from build123d import *

# Parameters (mm, degrees)
EXTRUDE_1_DEPTH = 35
FILLET_1_R      = 3


with BuildPart() as part:
    # 스케치1 → 보스-돌출1 (new body)
    with BuildSketch(Plane.XY):
        with BuildLine():
            Line((0, 0), (52.851450041, 0))
            Line((52.851450041, 0), (25.161162212, 33))
            ThreePointArc((25.161162212, 33), (20.274657466, 29.059278699), (15.388152719, 33))
            Line((15.388152719, 33), (0, 0))
        make_face()
    extrude(amount=EXTRUDE_1_DEPTH)

    # 필렛1
    fillet_1_edges = [part.edges().sort_by_distance(p)[0] for p in [
        (52.851450041, 0, 17.5),
        (0, 0, 17.5),
    ]]
    fillet(fillet_1_edges, radius=FILLET_1_R)


solid = part.part
Input: part model. Units: mm. Frame: model coordinates. Give positions to 0.01 mm unless a question says otherwise; leave off trailing zeros. Write each loop counter-clockwise with the first axis right and the second up, starting at its lowest first coordinate (ties: lowest second). Pieces come first, ordered by that corner, then holes.
Q1. Section C-C, the plane x = 32. Output: boundary loops of the cut face in (y, z), plus the area to 3 significant figures.
Q2. Pull-direction query (X, two-part tool) for faces 1 (the face through (20.37, 29.06, 17.26)), 2 (the face through (2.202, 1.353, 17.745)), 3 (the face through (25, 13, 35)); classes: pulls with the +X half, pulls with the -X half, needs draft (parallel to the pull), parting line crosses it, or undercut.
Q3. Material intervals for probe 1 along Y at (x, z) = (20, 22); probe 2 along X at (y, z) = (18.5, 4.5); probe 3 along Y at (x, z) = (32.5, 15), sorted ascending.
Q4. First-contact query: P1, Ø1, axis at y = 11.5, z = 18, coming from the -X side; P2, Ø6, axis at y = 29.5, z = 23.5, coming from the -X side; P3, Ø1.5, axis at y = 13, z = 18.5, coming from the -X side. Flat tips, straight axial feed; report the tip coordinate or a pass-through.
Q5. Section B-B, the plane y = 31. Output: boundary loops of the cut face in (x, z), plus the area to 3 significant figures.
Q6. Section A-A, the plane z = 10. Output: boundary loops of the cut face in (x, y), plus the area to 3 significant figures.
Q7. Section D-D, the plane y = 13. Output: boundary loops of the cut face in (x, z), plus the area to 3 significant figures.
Filled in:
1. outline: (0, 0) - (24.85, 0) - (24.85, 35) - (0, 35) - close
1. area: 870 mm2
2. face 1: undercut
2. face 2: pulls with the -X half
2. face 3: needs draft
3. probe 1: y = 0 to 29.07
3. probe 2: x = 8.63 to 37.33
3. probe 3: y = 0 to 24.25
4. P1: stops at x = 5.13
4. P2: stops at x = 12.36
4. P3: stops at x = 5.71
5. outline: (14.46, 0) - (16.32, 0) - (16.32, 35) - (14.46, 35) - close; (24.23, 0) - (26.84, 0) - (26.84, 35) - (24.23, 35) - close
5. area: 157 mm2
6. outline: (1.99, 4.27) arc R3 ccw to (4.71, 0) - (46.42, 0) arc R3 ccw to (48.72, 4.93) - (25.16, 33) arc R5 cw to (15.39, 33) - close
6. area: 990 mm2
7. outline: (6.06, 0) - (41.94, 0) - (41.94, 35) - (6.06, 35) - close
7. area: 1,260 mm2
